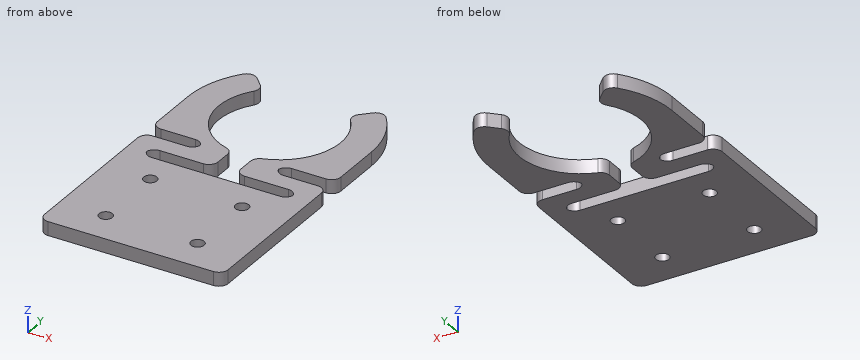
```python
from build123d import *

# Parameters (mm, degrees)
SKETCH_1_R          = 1.45
EXTRUDE_1_DEPTH     = 3
SKETCH_2_W          = 5
SKETCH_2_H          = 25
CUT_EXTRUDE_1_DEPTH = 49.554383298
SKETCH_3_W          = 11.5
SKETCH_3_H          = 3
SKETCH_3_W_2        = 13.5
CUT_EXTRUDE_2_DEPTH = 49.554383298
FILLET_1_R          = 2


with BuildPart() as part:
    # 草图1 → 凸台-拉伸1 (new body)
    with BuildSketch(Plane.XY):
        with BuildLine():
            Line((-9.40452019, 39.40452019), (-14.142135624, 44.142135624))
            ThreePointArc((-14.142135624, 44.142135624), (-18.47759065, 37.653668647), (-20, 30))
            Line((-20, 30), (-20, -23.5))
            Line((-20, -23.5), (20, -23.5))
            Line((20, -23.5), (20, 30))
            ThreePointArc((20, 30), (18.47759065, 37.653668647), (14.142135624, 44.142135624))
            Line((14.142135624, 44.142135624), (9.40452019, 39.40452019))
            ThreePointArc((9.40452019, 39.40452019), (0, 16.7), (-9.40452019, 39.40452019))
        make_face()
        with Locations((-10, 0)):
            Circle(SKETCH_1_R, mode=Mode.SUBTRACT)
        with Locations((10, 0)):
            Circle(SKETCH_1_R, mode=Mode.SUBTRACT)
        with Locations((-10, -16)):
            Circle(SKETCH_1_R, mode=Mode.SUBTRACT)
        with Locations((10, -16)):
            Circle(SKETCH_1_R, mode=Mode.SUBTRACT)
    extrude(amount=EXTRUDE_1_DEPTH)

    # 草图2 → 切除-拉伸1 (cut, through all)
    with BuildSketch(Plane.XY.offset(3)):
        with Locations((0, 19.5)):
            Rectangle(SKETCH_2_W, SKETCH_2_H)
    extrude(amount=-CUT_EXTRUDE_1_DEPTH, mode=Mode.SUBTRACT)

    # 草图3 → 切除-拉伸2 (cut, through all)
    with BuildSketch(Plane.XY.offset(3)):
        with Locations((-14.25, 15.5)):
            Rectangle(SKETCH_3_W, SKETCH_3_H)
        with Locations((-9.25, 8.5)):
            Rectangle(SKETCH_3_W_2, SKETCH_3_H)
        with Locations((9.25, 8.5)):
            Rectangle(SKETCH_3_W_2, SKETCH_3_H)
        with Locations((14.25, 15.5)):
            Rectangle(SKETCH_3_W, SKETCH_3_H)
    extrude(amount=-CUT_EXTRUDE_2_DEPTH, mode=Mode.SUBTRACT)

    # 圆角1
    # the kernel refuses this fillet: 2 mm, written as the material it adds along each edge
    with BuildSketch(Plane(origin=(8.5, 17, 3), x_dir=(1, 0, 0), z_dir=(0, 0, -1)), Plane(origin=(8.5, 14, 3), x_dir=(0, 1, 0), z_dir=(0, 0, -1)), Plane(origin=(-8.5, 14, 3), x_dir=(-1, 0, 0), z_dir=(0, 0, -1)), Plane(origin=(-8.5, 17, 3), x_dir=(0, -1, 0), z_dir=(0, 0, -1)), Plane(origin=(-16, 10, 3), x_dir=(1, 0, 0), z_dir=(0, 0, -1)), Plane(origin=(-16, 7, 3), x_dir=(0, 1, 0), z_dir=(0, 0, -1)), Plane(origin=(16, 7, 3), x_dir=(-1, 0, 0), z_dir=(0, 0, -1)), Plane(origin=(16, 10, 3), x_dir=(0, -1, 0), z_dir=(0, 0, -1))) as fillet_1_piece_1:
        with BuildLine():
            CenterArc((FILLET_1_R, FILLET_1_R), FILLET_1_R, 180, 90)
            Line((0, FILLET_1_R), (0, 0))
            Line((0, 0), (FILLET_1_R, 0))
        make_face()
    extrude(amount=3)
    # the kernel refuses this fillet: 2 mm, written as the material it takes off along each edge
    with BuildSketch(Plane(origin=(20, 14, 8), x_dir=(0, -1, 0), z_dir=(0, 0, -1)), Plane(origin=(-20, 14, 8), x_dir=(1, 0, 0), z_dir=(0, 0, -1)), Plane(origin=(-20, 17, 8), x_dir=(0, 1, 0), z_dir=(0, 0, -1)), Plane(origin=(-2.5, 10, 8), x_dir=(-1, 0, 0), z_dir=(0, 0, -1)), Plane(origin=(2.5, 10, 8), x_dir=(0, 1, 0), z_dir=(0, 0, -1)), Plane(origin=(20, 17, 8), x_dir=(-1, 0, 0), z_dir=(0, 0, -1))) as fillet_1_2_piece_1:
        with BuildLine():
            CenterArc((FILLET_1_R, FILLET_1_R), FILLET_1_R, 180, 90)
            Line((0, FILLET_1_R), (0, 0))
            Line((0, 0), (FILLET_1_R, 0))
        make_face()
    extrude(amount=13, mode=Mode.SUBTRACT)
    with BuildSketch(Plane(origin=(20, -23.5, -5), x_dir=(-1, 0, 0), z_dir=(0, 0, 1)), Plane(origin=(-20, -23.5, -5), x_dir=(0, 1, 0), z_dir=(0, 0, 1))) as fillet_1_2_piece_2:
        with BuildLine():
            CenterArc((FILLET_1_R, -FILLET_1_R), FILLET_1_R, 90, 90)
            Line((0, -FILLET_1_R), (0, 0))
            Line((0, 0), (FILLET_1_R, 0))
        make_face()
    extrude(amount=13, mode=Mode.SUBTRACT)
    with BuildSketch(Plane(origin=(-14.142135624, 44.142135624, -5.56417559), x_dir=(0.7071067811865518, -0.7071067811865434, 0), z_dir=(0, 0, 1))) as fillet_1_2_piece_3:
        with BuildLine():
            CenterArc((2.11145618, -2), FILLET_1_R, 90, 96.379370208)
            ThreePointArc((0.1238402, -2.222222222), (0.03098405, -1.112835118), (0, 0))
            Line((0, 0), (2.11145618, 0))
        make_face()
    extrude(amount=14.128351181, mode=Mode.SUBTRACT)
    with BuildSketch(Plane(origin=(-2.5, 16.937075366, 6.900861235), x_dir=(0, -1, 0), z_dir=(0, 0, -1))) as fillet_1_2_piece_4:
        with BuildLine():
            CenterArc((1.560344494, 2), FILLET_1_R, 197.104635177, 72.895364823)
            ThreePointArc((-0.351193954, 1.411764706), (-0.156279677, 0.71068777), (0, 0))
            Line((0, 0), (1.560344494, 0))
        make_face()
    extrude(amount=10.80172247, mode=Mode.SUBTRACT)
    with BuildSketch(Plane(origin=(2.5, 16.937075366, 6.900861235), x_dir=(0.9704244328417233, 0.2414050955216561, 0), z_dir=(0, 0, -1))) as fillet_1_2_piece_5:
        with BuildLine():
            CenterArc((1.564173754, 1.997006612), FILLET_1_R, 193.969485078, 72.895364823)
            Line((-0.376675112, 1.514196421), (0, 0))
            ThreePointArc((0, 0), (0.727395487, 0.019906032), (1.454790974, 0))
        make_face()
    extrude(amount=10.80172247, mode=Mode.SUBTRACT)
    with BuildSketch(Plane(origin=(9.40452019, 39.40452019, -4.671794525), x_dir=(0.6592727226844873, -0.7519039015221182, 0), z_dir=(0, 0, 1))) as fillet_1_2_piece_6:
        with BuildLine():
            CenterArc((1.873303853, 1.995705121), FILLET_1_R, 183.755569948, 82.488860105)
            Line((-0.122401268, 1.864704851), (0, 0))
            ThreePointArc((0, 0), (0.871151792, 0.028560946), (1.742303583, 0))
        make_face()
    extrude(amount=12.34358905, mode=Mode.SUBTRACT)
    with BuildSketch(Plane(origin=(14.142135624, 44.142135624, -5.56417559), x_dir=(-0.7071067811865467, -0.7071067811865483, 0), z_dir=(0, 0, 1))) as fillet_1_2_piece_7:
        with BuildLine():
            CenterArc((2.11145618, 2), FILLET_1_R, 173.620629792, 96.379370208)
            ThreePointArc((0.1238402, 2.222222222), (0.03098405, 1.112835118), (0, 0))
            Line((0, 0), (2.11145618, 0))
        make_face()
    extrude(amount=14.128351181, mode=Mode.SUBTRACT)
    with BuildSketch(Plane(origin=(-9.40452019, 39.40452019, -4.671794525), x_dir=(-0.659272722684483, -0.7519039015221219, 0), z_dir=(0, 0, 1))) as fillet_1_2_piece_8:
        with BuildLine():
            CenterArc((1.873303853, -1.995705121), FILLET_1_R, 93.755569948, 82.488860105)
            Line((-0.122401268, -1.864704851), (0, 0))
            ThreePointArc((0, 0), (0.871151792, -0.028560946), (1.742303583, 0))
        make_face()
    extrude(amount=12.34358905, mode=Mode.SUBTRACT)


solid = part.part
```
Here's how the part is built. I have some questions about the finished solid (model axes, mm). Give positions to 0.01 mm unless a question says otherwise; leave off trailing zeros. Order: outer loops, then holes, each group sorted by start corner. A loop starts at its lowest first (then second) coordinate and runs counter-clockwise, first axis right, second up. Notation, with made-up numbers: M 71,68 L 79,68 A21 ccw 79,74 Z; hole C 26.5,77 d8. An arc over 180 degrees is marked long. Use a Markdown table: item, result. Add a question column.
1. For pin 1 Ø1.5 at (x, z) = (-3.5, 1) entering from +Y; pin 2 Ø4.5 at (x, y) = (10, -16) entering from +Z; pin 3 Ø1.5 at (x, z) = (15.5, 2) entering from +Y; pin 4 Ø2.5 at (x, y) = (-10, -16) entering from +Z, each with a flat end and sliding along its axis, tell me the tip position at first contact or that it passes through.
2. Suppose I cut it at B-B (x = 5.5). List the corners of the cut face in (y, z) for me.
3. I need wall thicknesses on probe 1 along X at (y, z) = (-0.5, 0.45); probe 2 along X at (y, z) = (12, 1.5); probe 3 along Y at (x, z) = (10, 1.3). Which ranges of each line are inside material? Lowest first, please. Write a range as from..to.
4. Suppose I cut it at C-C (y = 22.5). List the corners of the cut face in (x, z) for me.
5. Suppose I cut it at D-D (z = 2.4). Give the number of separate pieces and of enclosed holes in the cut face, and give its area (3 significant figures).
6. Suppose I cut it at A-A (y = -16). List the corners of the cut face in (x, z) for me, and give its area (3 significant figures).
Results list:
| question | item | result |
|---|---|---|
| 1 | pin 1 | stops at y = 17.4 |
| 1 | pin 2 | stops at z = 3 |
| 1 | pin 3 | stops at y = 43.11 |
| 1 | pin 4 | passes through |
| 2 | outline | M -23.5,0 L 7,0 L 7,3 L -23.5,3 Z; M 10,0 L 17.89,0 L 17.89,3 L 10,3 Z |
| 3 | probe 1 | x = -20..-11.36, -8.64..8.64, 11.36..20 |
| 3 | probe 2 | x = -20..-2.5, 2.5..20 |
| 3 | probe 3 | y = -23.5..-17.45, -14.55..-1.45, 1.45..7, 10..14.06, 16.94..21.23 |
| 4 | outline | M -20,0 L -10.98,0 L -10.98,3 L -20,3 Z; M 10.98,0 L 20,0 L 20,3 L 10.98,3 Z |
| 5 | separate pieces | 1 |
| 5 | enclosed holes | 4 |
| 5 | area | 1,810 mm² |
| 6 | outline | M -20,0 L -11.45,0 L -11.45,3 L -20,3 Z; M -8.55,0 L 8.55,0 L 8.55,3 L -8.55,3 Z; M 11.45,0 L 20,0 L 20,3 L 11.45,3 Z |
| 6 | area | 103 mm² |
